For this review, take the finished solid that the model builds, in its own axes (mm). Face numbers are marked on the shaded views. A direction names the side the tool comes from. Round coordinates to 2 decimals unless told otherwise and drop trailing zeros. Loops run counter-clockwise (first coordinate to the right, second up) from the corner with the lowest first, then second, coordinate; pieces in that order, holes last.
1) Take a section at A-A (y = 3.25). State the section outline as (x, z) points, then the cut area to 3 significant figures.
2) Insertion check: pin 1 (3 mm diameter, centred on y = 14, z = 4.5, fed in from +X); pin 2 (1.5 mm diameter, centred on x = 21, y = 3, fed in from -Z); pin 3 (4 mm diameter, centred on y = 4.5, z = -5, fed in from -X); pin 4 (4 mm diameter, centred on x = 24.5, z = -1, fed in from +Y). Each pin has a flat end and moves straight along its axis. Give the tip position at first contact, or say it passes through.
3) Take a section at D-D (y = 14.25). State the section outline as (x, z) points, then the cut area to 3 significant figures.
4) Wall thickness on L1, parallel to X at y = 13.25, z = 24.5; L2, parallel to Z at x = 33, y = 11; L3, parallel to Y at x = -17, z = -14: over which ranges is each line inside the solid? List them lowest first.
5) Tool access review of the marked faces 1 and 2: name each direction out of +Z, -Z, +X, -X, +Y, -Y from which nothing blocks a thin tool from reaching the whole face with its end or side.
6) Take a section at B-B (x = 26.5). State the section outline as (y, z) points.
7) Take a section at C-C (z = -3.5). State the section outline as (x, y) points.
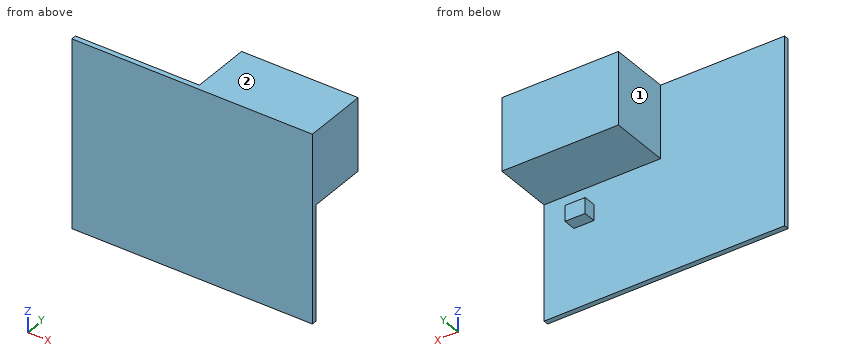
```python
from build123d import *

# Parameters (mm, degrees)
SKETCH1_W           = 76.5048
SKETCH1_H           = 59.6646
BOSS_EXTRUDE1_DEPTH = 1.62
SKETCH2_W           = 37.084
SKETCH2_H           = 23.114
BOSS_EXTRUDE2_DEPTH = 19.05
SKETCH3_W           = 6.362801742
SKETCH3_H           = 5.001103528
BOSS_EXTRUDE3_DEPTH = 4


with BuildPart() as part:
    # Sketch1 → Boss-Extrude1 (new body)
    with BuildSketch(Plane(origin=(0, 0, 0), x_dir=(1, 0, 0), z_dir=(0, 1, 0))):
        Rectangle(SKETCH1_W, SKETCH1_H)
    extrude(amount=BOSS_EXTRUDE1_DEPTH)

    # Sketch2 → Boss-Extrude2 (add)
    with BuildSketch(Plane(origin=(0, 1.62, 0), x_dir=(1, 0, 0), z_dir=(0, 1, 0))):
        with Locations((19.7104, -18.2753)):
            Rectangle(SKETCH2_W, SKETCH2_H)
    extrude(amount=BOSS_EXTRUDE2_DEPTH)

    # Sketch3 → Boss-Extrude3 (add)
    with BuildSketch(Plane(origin=(0, 1.62, 0), x_dir=(1, 0, 0), z_dir=(0, 1, 0))):
        with Locations((25.5524, 1.9177)):
            Rectangle(SKETCH3_W, SKETCH3_H)
    extrude(amount=BOSS_EXTRUDE3_DEPTH)


solid = part.part
```
Response:
1. outline: (1.17, 6.72) - (38.25, 6.72) - (38.25, 29.83) - (1.17, 29.83) - close; (22.37, -4.42) - (28.73, -4.42) - (28.73, 0.58) - (22.37, 0.58) - close
1. area: 889 mm2
2. pin 1: passes through
2. pin 2: stops at z = 6.72
2. pin 3: stops at x = 22.37
2. pin 4: stops at y = 5.62
3. outline: (1.17, 6.72) - (38.25, 6.72) - (38.25, 29.83) - (1.17, 29.83) - close
3. area: 857 mm2
4. L1: x = 1.17 to 38.25
4. L2: z = 6.72 to 29.83
4. L3: y = 0 to 1.62
5. face 1: +Z, -Z, -X, +Y
5. face 2: +Z, +X, -X, +Y, -Y
6. outline: (0, -29.83) - (1.62, -29.83) - (1.62, -4.42) - (5.62, -4.42) - (5.62, 0.58) - (1.62, 0.58) - (1.62, 6.72) - (20.67, 6.72) - (20.67, 29.83) - (0, 29.83) - close
7. outline: (-38.25, 0) - (38.25, 0) - (38.25, 1.62) - (28.73, 1.62) - (28.73, 5.62) - (22.37, 5.62) - (22.37, 1.62) - (-38.25, 1.62) - close
